from build123d import *

# Parameters (mm, degrees)
SKETCH1_W                       = 20.480821918
SKETCH1_H                       = 31.9
SKETCH1_R                       = 2.45
BOSS_EXTRUDE1_DEPTH             = 7.5
SKETCH2_W                       = 18.980821918
SKETCH2_H                       = 9.35
CUT_EXTRUDE1_DEPTH              = 6.2
CUT_EXTRUDE2_REACH              = 22.384
SKETCH5_W                       = 5.480821918
SKETCH5_H                       = 31.9
SKETCH3_R                       = 3
SKETCH3_R_2                     = 1.55
BOSS_EXTRUDE4_DEPTH             = 6.2
SKETCH6_W                       = 1.5
SKETCH6_H                       = 15.5
CUT_EXTRUDE3_DEPTH              = 6.2
SKETCH7_W                       = 1.5
SKETCH7_H                       = 18.7
BOSS_EXTRUDE5_DEPTH             = 6.2
FILLET1_R                       = 3
SKETCH8_W                       = 6
SKETCH8_H                       = 4
CUT_EXTRUDE4_DEPTH              = 7.5
FILLET2_R                       = 3
BOSS_EXTRUDE6_REACH             = 21.943
BOSS_EXTRUDE6_DIRECTION_2_REACH = 21.943
SKETCH10_R                      = 3.25
CUT_EXTRUDE6_DEPTH              = 4.5
FILLET3_R                       = 1.5
SKETCH12_W                      = 1.5
SKETCH12_H                      = 15.5
BOSS_EXTRUDE7_DEPTH             = 6.2


with BuildPart() as part:
    # Sketch1 → Boss-Extrude1 (new body)
    with BuildSketch(Plane.XY):
        Rectangle(SKETCH1_W, SKETCH1_H)
        with Locations((6.290410959, 12)):
            Circle(SKETCH1_R, mode=Mode.SUBTRACT)
        with Locations((6.290410959, -12)):
            Circle(SKETCH1_R, mode=Mode.SUBTRACT)
    extrude(amount=BOSS_EXTRUDE1_DEPTH)

    # Sketch2 → Cut-Extrude1 (cut)
    with BuildSketch(Plane.XY.offset(7.5)):
        with Locations((-0.75, 4.675)):
            Rectangle(SKETCH2_W, SKETCH2_H)
        with Locations((-0.75, -4.675)):
            Rectangle(SKETCH2_W, SKETCH2_H)
    extrude(amount=-CUT_EXTRUDE1_DEPTH, mode=Mode.SUBTRACT)

    # Cut-Extrude2: up to this face of the body (flat: up to its plane)
    cut_extrude2_end = Plane(part.part.faces().sort_by_distance((-0.385368256, 0, 0))[0])
    # Sketch5 → Cut-Extrude2 (cut, up to the picked face)
    with BuildSketch(Plane.XY.offset(7.5), mode=Mode.PRIVATE) as cut_extrude2_sk1:
        with Locations((-7.5, 0)):
            Rectangle(SKETCH5_W, SKETCH5_H)
    cut_extrude2_tool1 = split(extrude(cut_extrude2_sk1.sketch, amount=-CUT_EXTRUDE2_REACH, mode=Mode.PRIVATE), bisect_by=cut_extrude2_end, keep=Keep.BOTH, mode=Mode.PRIVATE)
    add(cut_extrude2_tool1.solids().sort_by(Axis((-7.5, 0, 7.5), (0, 0, -1)))[0], mode=Mode.SUBTRACT)

    # Sketch3 → Boss-Extrude4 (add)
    # profile 1 of 2: a face of its own
    with BuildSketch(Plane.XY.offset(1.3)):
        with Locations(Location((-1.259589041, 5, 0), (0, 0, 180))):
            Circle(SKETCH3_R)
        with Locations(Location((-1.259589041, 5, 0), (0, 0, 180))):
            Circle(SKETCH3_R_2, mode=Mode.SUBTRACT)
    # profile 2 of 2: a face of its own
    with BuildSketch(Plane.XY.offset(1.3)):
        with Locations(Location((-1.259589041, -5, 0), (0, 0, 180))):
            Circle(SKETCH3_R)
        with Locations(Location((-1.259589041, -5, 0), (0, 0, 180))):
            Circle(SKETCH3_R_2, mode=Mode.SUBTRACT)
    extrude(amount=BOSS_EXTRUDE4_DEPTH)

    # Sketch6 → Cut-Extrude3 (cut)
    with BuildSketch(Plane.XY.offset(7.5)):
        with Locations((9.490410959, 0)):
            Rectangle(SKETCH6_W, SKETCH6_H)
    extrude(amount=-CUT_EXTRUDE3_DEPTH, mode=Mode.SUBTRACT)

    # Sketch7 → Boss-Extrude5 (add)
    with BuildSketch(Plane.XY.offset(1.3)):
        with Locations((-4.009589041, 0)):
            Rectangle(SKETCH7_W, SKETCH7_H)
    extrude(amount=BOSS_EXTRUDE5_DEPTH)

    # Fillet1
    fillet1_edges = [part.edges().sort_by_distance(p)[0] for p in [
        (10.240410959, 15.95, 3.75),
        (10.240410959, -15.95, 3.75),
    ]]
    fillet(fillet1_edges, radius=FILLET1_R)

    # Sketch8 → Cut-Extrude4 (cut)
    with BuildSketch(Plane.XY.offset(7.5)):
        with Locations((-1.759589041, 13.95)):
            Rectangle(SKETCH8_W, SKETCH8_H)
        with Locations((-1.759589041, -13.95)):
            Rectangle(SKETCH8_W, SKETCH8_H)
    extrude(amount=-CUT_EXTRUDE4_DEPTH, mode=Mode.SUBTRACT)

    # Fillet2
    fillet2_edges = [part.edges().sort_by_distance(p)[0] for p in [
        (1.240410959, 15.95, 3.75),
        (-4.759589041, 11.95, 3.75),
        (1.240410959, -15.95, 3.75),
        (-4.759589041, -11.95, 3.75),
    ]]
    fillet(fillet2_edges, radius=FILLET2_R)

    # Boss-Extrude6: up to this face of the body (flat: up to its plane)
    boss_extrude6_end = Plane(part.part.faces().sort_by_distance((5.740410959, -15.597493262, 7.5))[0])
    # Sketch11 → Boss-Extrude6 (add, up to the picked face)
    with BuildSketch(Plane.XY.offset(1.3), mode=Mode.PRIVATE) as boss_extrude6_sk1:
        with BuildLine():
            Line((-3.259589041, 9.35), (-3.259589041, 7.236067977))
            ThreePointArc((-3.259589041, 7.236067977), (-1.735455251, 7.962018121), (-0.06063116, 7.75))
            Line((-0.06063116, 7.75), (8.740410959, 7.75))
            Line((8.740410959, 7.75), (8.740410959, 9.35))
            Line((8.740410959, 9.35), (-3.259589041, 9.35))
        make_face()
    boss_extrude6_tool1 = split(extrude(boss_extrude6_sk1.sketch, amount=BOSS_EXTRUDE6_REACH, mode=Mode.PRIVATE), bisect_by=boss_extrude6_end, keep=Keep.BOTH, mode=Mode.PRIVATE)
    # Sketch11 → Boss-Extrude6 (add, up to the picked face)
    with BuildSketch(Plane.XY.offset(1.3), mode=Mode.PRIVATE) as boss_extrude6_sk2:
        with BuildLine():
            Line((-3.259589041, -7.236067977), (-3.259589041, -9.35))
            Line((-3.259589041, -9.35), (8.740410959, -9.35))
            Line((8.740410959, -9.35), (8.740410959, -7.75))
            Line((8.740410959, -7.75), (-0.06063116, -7.75))
            ThreePointArc((-0.06063116, -7.75), (-1.735455251, -7.962018121), (-3.259589041, -7.236067977))
        make_face()
    boss_extrude6_tool2 = split(extrude(boss_extrude6_sk2.sketch, amount=BOSS_EXTRUDE6_REACH, mode=Mode.PRIVATE), bisect_by=boss_extrude6_end, keep=Keep.BOTH, mode=Mode.PRIVATE)
    add(boss_extrude6_tool1.solids().sort_by(Axis((2.770321, 8.555653, 1.3), (0, 0, 1)))[0])
    add(boss_extrude6_tool2.solids().sort_by(Axis((2.770321, -8.555653, 1.3), (0, 0, 1)))[0])

    # Boss-Extrude6 direction 2: up to this face of the body (flat: up to its plane)
    boss_extrude6_direction_2_end = Plane(part.part.faces().sort_by_distance((2.964227546, 0, 0))[0])
    # Sketch11 → Boss-Extrude6 direction 2 (add, up to the picked face)
    with BuildSketch(Plane.XY.offset(1.3), mode=Mode.PRIVATE) as boss_extrude6_direction_2_sk1:
        with BuildLine():
            Line((-3.259589041, 9.35), (-3.259589041, 7.236067977))
            ThreePointArc((-3.259589041, 7.236067977), (-1.735455251, 7.962018121), (-0.06063116, 7.75))
            Line((-0.06063116, 7.75), (8.740410959, 7.75))
            Line((8.740410959, 7.75), (8.740410959, 9.35))
            Line((8.740410959, 9.35), (-3.259589041, 9.35))
        make_face()
    boss_extrude6_direction_2_tool1 = split(extrude(boss_extrude6_direction_2_sk1.sketch, amount=-BOSS_EXTRUDE6_DIRECTION_2_REACH, mode=Mode.PRIVATE), bisect_by=boss_extrude6_direction_2_end, keep=Keep.BOTH, mode=Mode.PRIVATE)
    # Sketch11 → Boss-Extrude6 direction 2 (add, up to the picked face)
    with BuildSketch(Plane.XY.offset(1.3), mode=Mode.PRIVATE) as boss_extrude6_direction_2_sk2:
        with BuildLine():
            Line((-3.259589041, -7.236067977), (-3.259589041, -9.35))
            Line((-3.259589041, -9.35), (8.740410959, -9.35))
            Line((8.740410959, -9.35), (8.740410959, -7.75))
            Line((8.740410959, -7.75), (-0.06063116, -7.75))
            ThreePointArc((-0.06063116, -7.75), (-1.735455251, -7.962018121), (-3.259589041, -7.236067977))
        make_face()
    boss_extrude6_direction_2_tool2 = split(extrude(boss_extrude6_direction_2_sk2.sketch, amount=-BOSS_EXTRUDE6_DIRECTION_2_REACH, mode=Mode.PRIVATE), bisect_by=boss_extrude6_direction_2_end, keep=Keep.BOTH, mode=Mode.PRIVATE)
    add(boss_extrude6_direction_2_tool1.solids().sort_by(Axis((2.770321, 8.555653, 1.3), (0, 0, -1)))[0])
    add(boss_extrude6_direction_2_tool2.solids().sort_by(Axis((2.770321, -8.555653, 1.3), (0, 0, -1)))[0])

    # Sketch10 → Cut-Extrude6 (cut)
    with BuildSketch(Plane(origin=(0, 0, 0), x_dir=(-1, 0, 0), z_dir=(0, 0, -1))):
        with Locations((-6.290410959, 12)):
            Circle(SKETCH10_R)
        with Locations((-6.290410959, -12)):
            Circle(SKETCH10_R)
    extrude(amount=-CUT_EXTRUDE6_DEPTH, mode=Mode.SUBTRACT)

    # Fillet3
    fillet3_edges = [part.edges().sort_by_distance(p)[0] for p in [
        (1.265413056, 3.380010984, 1.3),
        (1.265413056, -3.380010984, 1.3),
    ]]
    fillet(fillet3_edges, radius=FILLET3_R)

    # Sketch12 → Boss-Extrude7 (add)
    with BuildSketch(Plane.XY.offset(1.3)):
        with Locations((9.490410959, 0)):
            Rectangle(SKETCH12_W, SKETCH12_H)
    extrude(amount=BOSS_EXTRUDE7_DEPTH)


solid = part.part
Geometry: final body of the model. Coordinates: model frame, mm. A direction names the side the tool comes from. Give positions to 0.01 mm unless a question says otherwise; leave off trailing zeros. Order: outer loops, then holes, each group sorted by start corner. A loop starts at its lowest first (then second) coordinate and runs counter-clockwise, first axis right, second up. Notation, with made-up numbers: (3.25, -2.75) -> (25.25, -2.75) arc R23 ccw to (25.25, 8.25) -> close; hole circle Ø2 at (77.25, -27). An arc over 180 degrees is marked (long way). Put each result on its own line as item: value.
Q1. Material intervals for L1, parallel to X at y = 5, z = 5.75; L2, parallel to X at y = -4, z = 3; L3, parallel to X at y = 0, z = 6, sorted ascending.
Here are the results:
L1: x = -4.76 to -2.81, 0.29 to 1.74, 8.74 to 10.24
L2: x = -4.76 to -2.44, -0.08 to 1.57, 8.74 to 10.24
L3: x = -4.76 to -3.26, 8.74 to 10.24
Q2. Draft query along Y for faces 5 (the face through (10.24, 0, 4)), 6 (the face through (-3.86, -11.09, 3.7)), 7 (the face through (8.74, 0, 4)). Return one class per face: released by +Y, released by -Y, zero draft, split by the parting line, or undercut.
Here are the results:
face 5: zero draft
face 6: released by -Y
face 7: undercut
Q3. Section B-B, the plane z = 4. Return loops of the section in (x, y).
Here are the results:
outline: (-4.76, -8.95) arc R3 ccw to (-1.76, -11.95) -> (1.24, -11.95) -> (1.24, -12.95) arc R3 ccw to (4.24, -15.95) -> (7.24, -15.95) arc R3 ccw to (10.24, -12.95) -> (10.24, 12.95) arc R3 ccw to (7.24, 15.95) -> (4.24, 15.95) arc R3 ccw to (1.24, 12.95) -> (1.24, 11.95) -> (-1.76, 11.95) arc R3 ccw to (-4.76, 8.95) -> close; hole (-3.26, -2.76) arc R3 cw (long way) to (-0.06, -7.75) -> (8.74, -7.75) -> (8.74, 7.75) -> (-0.06, 7.75) arc R3 cw (long way) to (-3.26, 2.76) -> close; hole circle Ø3.1 at (-1.26, -5); hole circle Ø3.1 at (-1.26, 5); hole circle Ø6.5 at (6.29, -12); hole circle Ø6.5 at (6.29, 12)
Q4. Reachability of faces 1 (the face through (3.2, -11, 2.2)), 2 (the face through (9.385, 15.048, 3.802)), 3 (the face through (1.24, 12.4, 3.8)), 4 (the face through (0, -11.95, 4)) from +Z, -Z, +X, -X, +Y, -Y: full face, straight path, thin tool, end or side. Return the list, or none.
Here are the results:
face 1: -Z
face 2: +Z, -Z, +X, +Y
face 3: +Z, -Z, -X, +Y
face 4: +Z, -Z, -X, -Y
Q5. Section A-A, the plane y = 11. Return loops of the section in (x, z).
Here are the results:
outline: (-3.95, 0) -> (3.2, 0) -> (3.2, 4.5) -> (4.05, 4.5) -> (4.05, 7.5) -> (-3.95, 7.5) -> close; (8.53, 4.5) -> (9.38, 4.5) -> (9.38, 0) -> (10.24, 0) -> (10.24, 7.5) -> (8.53, 7.5) -> close
Q6. Section C-C, the plane y = 5. Return loops of the section in (x, z), then the cut area to 3 significant figures.
Here are the results:
outline: (-4.76, 0) -> (10.24, 0) -> (10.24, 7.5) -> (8.74, 7.5) -> (8.74, 1.3) -> (3.24, 1.3) arc R1.5 cw to (1.74, 2.8) -> (1.74, 7.5) -> (0.29, 7.5) -> (0.29, 1.3) -> (-2.81, 1.3) -> (-2.81, 7.5) -> (-4.76, 7.5) -> close
area: 50.4 mm^2
Q7. Section D-D, the plane x = 5.5. Return loops of the section in (y, z).
Here are the results:
outline: (-15.95, 0) -> (-15.15, 0) -> (-15.15, 4.5) -> (-14.32, 4.5) -> (-14.32, 7.5) -> (-15.95, 7.5) -> close; (-9.68, 4.5) -> (-8.85, 4.5) -> (-8.85, 0) -> (8.85, 0) -> (8.85, 4.5) -> (9.68, 4.5) -> (9.68, 7.5) -> (7.75, 7.5) -> (7.75, 1.3) -> (-7.75, 1.3) -> (-7.75, 7.5) -> (-9.68, 7.5) -> close; (14.32, 4.5) -> (15.15, 4.5) -> (15.15, 0) -> (15.95, 0) -> (15.95, 7.5) -> (14.32, 7.5) -> close
Q8. Pin query (flat end, axial travel): pin 1 (3 mm diameter, centred on x = 2, z = 4.5, fed in from +Y); pin 2 (2.5 mm diameter, centred on x = -1, y = -5, fed in from +Z); pin 3 (3.5 mm diameter, centred on x = -2, y = 4.5, fed in from +Z); pin 4 (1 mm diameter, centred on x = -2, z = 6.5, fed in from -Y). Return the tip coordinate at first contact, or that it passes through.
Here are the results:
pin 1: stops at y = 15.86
pin 2: stops at z = 1.3
pin 3: stops at z = 7.5
pin 4: stops at y = -11.95
